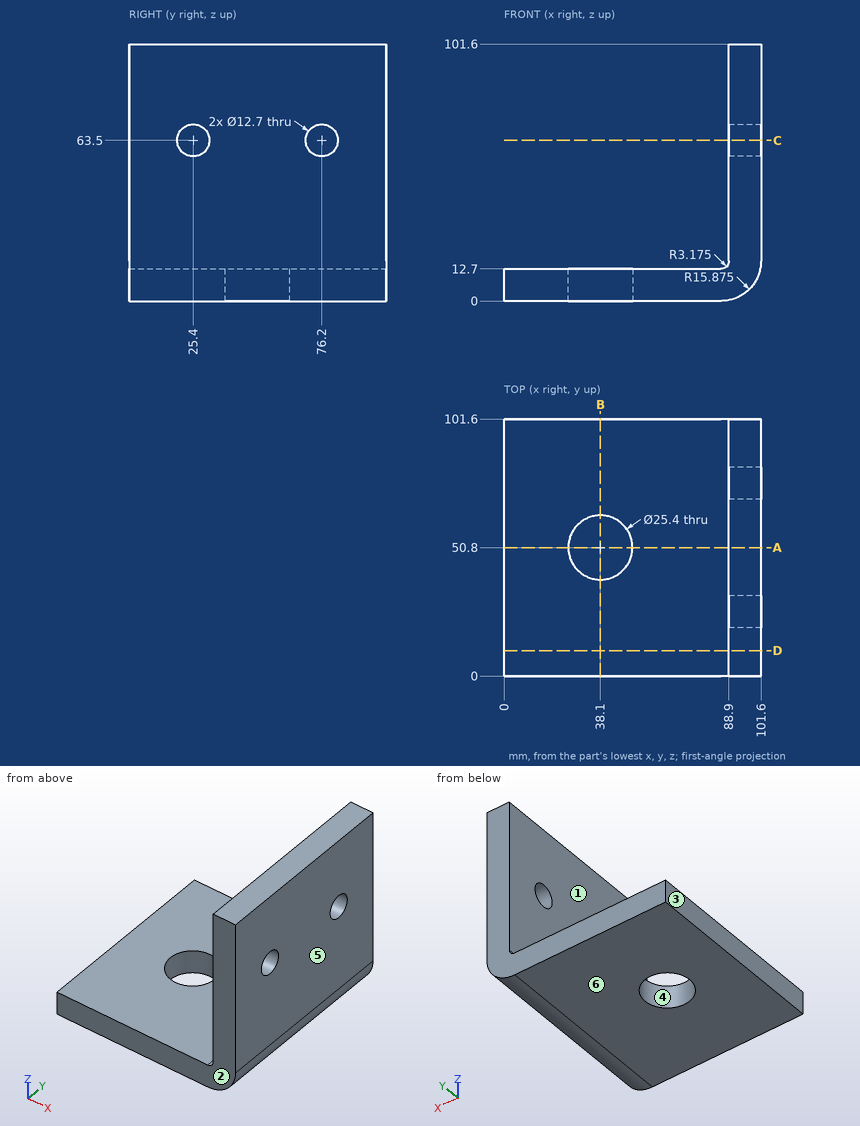
Job drawing, mm, ordinate dimensions from the low corner. One solid piece. A direction names the side the tool comes from. Coordinates: 2 decimals unless noted, no trailing zeros. Loops run counter-clockwise (first coordinate to the right, second up) from the corner with the lowest first, then second, coordinate; pieces in that order, holes last. Notation, with made-up numbers: (66, 1) - (92, 1) arc R32 cw to (92, 28) - close; hole circle Ø8 at (70.5, -29.75). An arc over 180 degrees is marked (long way). Answer as a JSON object with one key per item and string values. Group by question number.
(1) Tool access for the marked faces 1 and 2: list every direction of +Z, -Z, +X, -X, +Y, -Y with a clear straight run to the whole face (end or side of a thin tool).
(2) Flat gauge pin, fed straight in: pin 1 (12 mm diameter, centred on x = 37, z = 19, fed in from +Y). Where does the tip first touch, or does it go through?
(3) Probe line 1 along Y through (x, z) = (94, 63); line 2 along Y through (x, z) = (38.1, 9); line 3 along X through (y, z) = (64.5, 49). List the from-to ranges inside material, lowest first.
(4) Cut at C-C (z = 63.5). Give the cut face in (x, y), then the cut area to 3 significant figures.
(5) Cut at B-B (x = 38.1). Give the cut face in (y, z).
(6) Two-plate mould, pull along X, no slides. Class the marked faces 3, 4, 5 and 6: released by +X, released by -X, zero draft, split by the parting line, or undercut.
(7) Cut at A-A (y = 50.8). Give the cut face in (x, z) (3 decimals), then the cut area to 3 significant figures.
(8) Cut at D-D (y = 10). Give the cut face in (x, z) (3 decimals).
Geometry says:
{
 "1": {"face 1": "+Z, -X, +Y, -Y", "face 2": "+Z, -Z, +X, -X, -Y"},
 "2": {"pin 1": "passes through"},
 "3": {"line 1": "y = 0 to 19.07, 31.73 to 69.87, 82.53 to 101.6", "line 2": "y = 0 to 38.1, 63.5 to 101.6", "line 3": "x = 88.9 to 101.6"},
 "4": {"outline": "(88.9, 0) - (101.6, 0) - (101.6, 19.05) - (88.9, 19.05) - close; (88.9, 31.75) - (101.6, 31.75) - (101.6, 69.85) - (88.9, 69.85) - close; (88.9, 82.55) - (101.6, 82.55) - (101.6, 101.6) - (88.9, 101.6) - close", "area": "968 mm^2"},
 "5": {"outline": "(0, 0) - (38.1, 0) - (38.1, 12.7) - (0, 12.7) - close; (63.5, 0) - (101.6, 0) - (101.6, 12.7) - (63.5, 12.7) - close"},
 "6": {"face 3": "released by -X", "face 4": "undercut", "face 5": "released by +X", "face 6": "zero draft"},
 "7": {"outline": "(0, 0) - (25.4, 0) - (25.4, 12.7) - (0, 12.7) - close; (50.8, 0) - (85.725, 0) arc R15.875 ccw to (101.6, 15.875) - (101.6, 101.6) - (88.9, 101.6) - (88.9, 15.875) arc R3.175 cw to (85.725, 12.7) - (50.8, 12.7) - close", "area": "2,040 mm^2"},
 "8": {"outline": "(0, 0) - (85.725, 0) arc R15.875 ccw to (101.6, 15.875) - (101.6, 101.6) - (88.9, 101.6) - (88.9, 15.875) arc R3.175 cw to (85.725, 12.7) - (0, 12.7) - close"}
}
